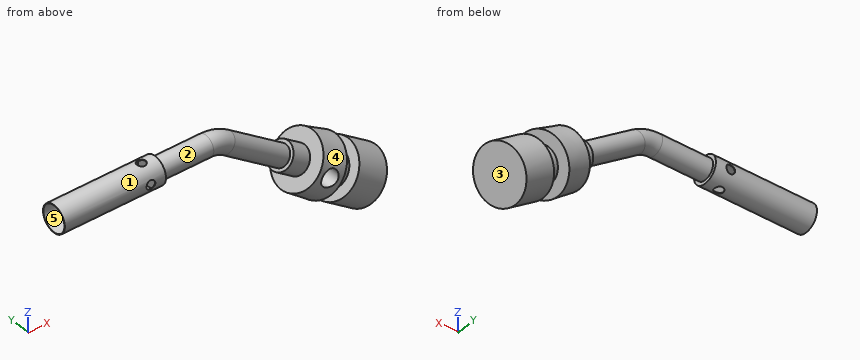
from build123d import *

# Parameters (mm, degrees)
F0_R           = 2.54
F1_DEPTH       = 19.05
F2_R           = 1.905
F5_R           = 2.54
F5_R_2         = 1.905
F6_DEPTH       = 3.81
F7_R           = 5.08
F7_R_2         = 2.54
F8_DEPTH       = 5.08
F8_TAPER       = -3
F9_R           = 3.175
F10_DEPTH      = 3.175
F11_R          = 5.08
F11_R_2        = 3.175
F12_DEPTH      = 6.35
F13_R          = 2.4436980308
F14_DEPTH      = 17.78
F15_R          = 0.8255
F16_DEPTH      = 23.1575077208
F16_DEPTH_BACK = 2.541
F17_R          = 0.8255
F18_DEPTH      = 5.3472316188
F18_DEPTH_BACK = 5.3472316188
F19_R          = 1.5875
F20_DEPTH      = 5.3472316188


with BuildPart() as f1:
    # F0 (on Right) → F1 (new body)
    with BuildSketch(Plane.YZ):
        Circle(F0_R)
    extrude(amount=F1_DEPTH)

    # F4: sweep along a path in F3
    with BuildLine(Plane.XZ) as f4_path:
        Line((19.05, 0), (28.575, 0))
        ThreePointArc((28.575, 0), (30.4844818269, -0.2938973627), (32.2172103708, -1.1483845188))
        Line((32.2172103708, -1.1483845188), (42.6204413333, -8.4328052604))
    # F2 (on face) → F4 (sweep)
    with BuildSketch(Plane.YZ.offset(19.05)):
        Circle(F2_R)
    sweep(path=f4_path.line)

    # F5 (on face) → F6 (join)
    with BuildSketch(Plane(origin=(32.5608678312, 0, -22.7993651061), x_dir=(0, 1, 0), z_dir=(0.8191520443, 0, -0.5735764364))):
        with Locations((0, 17.5383311875)):
            Circle(F5_R)
        with Locations((0, 17.5383311875)):
            Circle(F5_R_2, mode=Mode.SUBTRACT)
        with Locations((0, 17.5383311875)):
            Circle(F5_R_2)
    extrude(amount=F6_DEPTH)

    # F7 (on face) → F8 (join)
    with BuildSketch(Plane(origin=(35.68183712, 0, -24.9846913286), x_dir=(0, 1, 0), z_dir=(0.8191520443, 0, -0.5735764364))):
        with Locations((0, 17.5383311875)):
            Circle(F7_R)
        with Locations((0, 17.5383311875)):
            Circle(F7_R_2, mode=Mode.SUBTRACT)
        with Locations((0, 17.5383311875)):
            Circle(F7_R_2)
    extrude(amount=F8_DEPTH, taper=F8_TAPER)

    # F9 (on face) → F10 (join)
    with BuildSketch(Plane(origin=(39.843129505, 0, -27.8984596252), x_dir=(0, 1, 0), z_dir=(0.8191520443, 0, -0.5735764364))):
        with Locations((0, 17.5383311875)):
            Circle(F9_R)
    extrude(amount=F10_DEPTH)

    # F11 (on face) → F12 (join)
    with BuildSketch(Plane(origin=(42.4439372456, 0, -29.7195648107), x_dir=(0, 1, 0), z_dir=(0.8191520443, 0, -0.5735764364))):
        with Locations((0, 17.5383311875)):
            Circle(F11_R)
        with Locations((0, 17.5383311875)):
            Circle(F11_R_2, mode=Mode.SUBTRACT)
        with Locations((0, 17.5383311875)):
            Circle(F11_R_2)
    extrude(amount=F12_DEPTH)

    # F13 (on face) → F14 (cut)
    with BuildSketch(Plane(origin=(0, 0, 0), x_dir=(0, -1, 0), z_dir=(-1, 0, 0))):
        Circle(F13_R)
    extrude(amount=-F14_DEPTH, mode=Mode.SUBTRACT)

    # F15 (on Top) → F16 (cut, two sides)
    with BuildSketch(Plane.XY) as f16_sk:
        with Locations((16.4403449744, 0)):
            Circle(F15_R)
    extrude(amount=-F16_DEPTH, mode=Mode.SUBTRACT)
    extrude(f16_sk.sketch, amount=F16_DEPTH_BACK, mode=Mode.SUBTRACT)

    # F17 (on Front) → F18 (cut, two sides)
    with BuildSketch(Plane.XZ) as f18_sk:
        with Locations((16.2350572646, 0)):
            Circle(F17_R)
    extrude(amount=-F18_DEPTH, mode=Mode.SUBTRACT)
    extrude(f18_sk.sketch, amount=F18_DEPTH_BACK, mode=Mode.SUBTRACT)

    # F19 (on Front) → F20 (cut, through all)
    with BuildSketch(Plane.XZ):
        with Locations((47.8220568145, -12.0750156313)):
            Circle(F19_R)
    extrude(amount=F20_DEPTH, mode=Mode.SUBTRACT)


solid = f1.part
Input: part model. Units: mm. Frame: model coordinates. Face numbers are marked on the shaded views. A direction names the side the tool comes from. Coordinates: 2 decimals unless noted, no trailing zeros. Write each loop counter-clockwise with the first axis right and the second up, starting at its lowest first coordinate (ties: lowest second). Pieces come first, ordered by that corner, then holes. Notation, with made-up numbers: M 42.25,-12.5 L 77.25,-12.5 A9 cw 77.25,4.5 Z; hole C -34,31.5 d11. An arc over 180 degrees is marked long. Answer as a JSON object with one key per item and string values. Group by question number.
(1) Mould query, pull axis Y, two halves, no side actions, for the marked faces 3, 4 and 5. Classes: pulls with the +Y half, pulls with the -Y half, needs draft (parallel to the pull), parting line crosses it, or undercut.
(2) Section A-A on x = 12. Output: boundary loops of the cut face in (y, z).
(3) Set-up query: the marked faces 1 and 2. Return all of +Z, -Z, +X, -X, +Y, -Y with unobstructed straight access to the full face (end or side cutting, diameter ignored); none if empty.
(4) Ray query, line 1 along X through (y, z) = (2.4, 0); line 2 along X through (y, z) = (3.25, -14.5); line 3 along X through (y, z) = (0, -2.35). Return the intervals inside material, ascending. Write a range as [from, to].
(5) Contact query for flat-ended pins moving along their axis: P1, Ø5, axis at y = -1, z = -14, coming from the -X side; P2, Ø2, axis at x = 50.5, y = -4, coming from the -Z side; P3, Ø6, axis at y = 2, z = -17, coming from the -X side. Output: stop coordinate, or through.
Result set:
{
 "1": {"face 3": "needs draft", "face 4": "parting line crosses it", "face 5": "undercut"},
 "2": {"outline": "C 0,0 d5.08; hole C 0,0 d4.89"},
 "3": {"face 1": "-X", "face 2": "none"},
 "4": {"line 1": "x = [17.78, 19.05]", "line 2": "x = [44.35, 49.22], [53.1, 58.09]", "line 3": "x = [17.78, 19.05], [30.51, 37.25]"},
 "5": {"P1": "stops at x = 42.73", "P2": "stops at z = -19.19", "P3": "stops at x = 42.83"}
}
